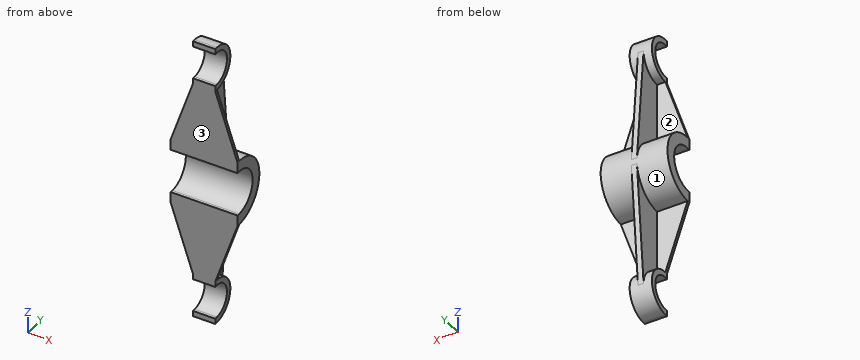
Autodesk Inventor part; units mm, degrees
ref_plane "YZ Plane" through (0, 0, 0) normal (1, 0, 0) x (0, 1, 0)
ref_plane "XZ Plane" through (0, 0, 0) normal (0, 1, 0) x (-1, 0, 0)
ref_plane "XY Plane" through (0, 0, 0) normal (0, 0, 1) x (1, 0, 0)
sketch "Boceto1" plane through (0, 0, 0) normal (1, 0, 0) x (0, 1, 0)
  arc A0 (0, -20) -> (0, 20) centre (0, 0) ccw
  arc A1 (0, -30) -> (0, 30) centre (0, 0) ccw
  line L0 (0, 0) -> (-5, 0) construction
  arc A2 (0, -125) -> (0, -95) centre (0, -110) ccw
  arc A3 (0, -130) -> (0, -90) centre (0, -110) ccw
  arc A4 (0, 95) -> (0, 125) centre (0, 110) ccw
  arc A5 (0, 90) -> (0, 130) centre (0, 110) ccw
  line L1 (0, 95) -> (-2.5, 95)
  line L2 (-2.5, 95) -> (-2.5, 90)
  line L3 (-2.5, 90) -> (0, 90)
  line L4 (0, 125) -> (-2.5, 125)
  line L5 (-2.5, 125) -> (-2.5, 130)
  line L6 (-2.5, 130) -> (0, 130)
  line L7 (0, -95) -> (-2.5, -95)
  line L8 (-2.5, -95) -> (-2.5, -90)
  line L9 (-2.5, -90) -> (0, -90)
  line L10 (0, -125) -> (-2.5, -125)
  line L11 (-2.5, -125) -> (-2.5, -130)
  line L12 (-2.5, -130) -> (0, -130)
  line L13 (0, 20) -> (-2.5, 20)
  line L14 (-2.5, 20) -> (-2.5, 30)
  line L15 (-2.5, 30) -> (0, 30)
  line L16 (0, -20) -> (-2.5, -20)
  line L17 (-2.5, -20) -> (-2.5, -30)
  line L18 (-2.5, -30) -> (0, -30)
  point P0 (0, 130)
  dimension "d0" = 20
  dimension "d1" = 30
  dimension "d2" = 5
  dimension "d3" = 15
  dimension "d5" = 20
  dimension "d6" = 110
  dimension "d7" = 2.5
  dimension "d8" = 5
  dimension "d9" = 5
  dimension "d10" = 10
  dimension "d11" = 10
  dimension "d16" = 2.5
extrude "Extrusión1" add sketch "Boceto1" along normal mid plane 60 contours A0 L13 L14 L15 A1 L18 L17 L16
extrude "Extrusión2" add sketch "Boceto1" along normal mid plane 20 contours A2 L7 L8 L9 A3 L12 L11 L10 | A4 L4 L5 L6 A5 L3 L2 L1
sketch "Boceto2" plane through (-30, -2.5, 20) normal (0, -1, 0) x (1, 0, 0)
  line L0 (40, 70) -> (20, 70)
  line L1 (40, 75) -> (40, 70)
  line L2 (60, 10) -> (40, 70)
  line L3 (0, 10) -> (60, 10)
  line L4 (20, 70) -> (0, 10)
  line L5 (60, -40) -> (60, -50)
  line L6 (60, -50) -> (40, -110)
  line L7 (20, -110) -> (0, -50)
  line L8 (0, -50) -> (60, -50)
  line L9 (60, -50) -> (0, -50)
  line L10 (60, 10) -> (60, 0)
  line L11 (60, 10) -> (0, 10)
  line L12 (20, -110) -> (40, -110)
  line L13 (40, -110) -> (20, -110)
  point P0 (30, -20)
extrude "Extrusión3" add sketch "Boceto2" against normal blind 2.5
sketch "Boceto3" plane through (0, 0, 0) normal (1, 0, 0) x (0, 1, 0)
  arc A0 (0, -130) -> (0, -90) centre (0, -110) ccw
  line L0 (20, -110) -> (29.8737, -2.7502)
  arc A1 (0, -30) -> (0, 30) centre (0, 0) ccw
  arc A2 (0, 90) -> (0, 130) centre (0, 110) ccw
  line L1 (20, 110) -> (29.9301, 2.1377)
  line L2 (0, -30) -> (0, -90)
  line L3 (0, 90) -> (0, 30)
  point P0 (29.8737, 2.7502)
extrude "Extrusión4" add sketch "Boceto3" along normal mid plane 5
properties part number "Pieza de practica 10"
Verification items for the finished model (mm, model axes). Face numbers are marked on the shaded views. A direction names the side the tool comes from. Coordinates: 2 decimals unless noted, no trailing zeros. Loops run counter-clockwise (first coordinate to the right, second up) from the corner with the lowest first, then second, coordinate; pieces in that order, holes last. Notation, with made-up numbers: (7, -39.75) -> (12, -39.75) arc R12 cw to (12, -21.75) -> close; hole circle Ø5 at (20.25, -31). An arc over 180 degrees is marked (long way). Answer in a Markdown table with one row per item.
1) Section check D-D (x = 6.5). Record the cut outline in (y, z), and give its area (3 significant figures).
The answers:
| item | result |
|---|---|
| outline | (-2.5, -130) -> (0, -130) arc R20 ccw to (0, -90) -> (0, -30) arc R30 ccw to (0, 30) -> (0, 90) arc R20 ccw to (0, 130) -> (-2.5, 130) -> (-2.5, 125) -> (0, 125) arc R15 cw to (0, 95) -> (-2.5, 95) -> (-2.5, 20) -> (0, 20) arc R20 cw to (0, -20) -> (-2.5, -20) -> (-2.5, -95) -> (0, -95) arc R15 cw to (0, -125) -> (-2.5, -125) -> close |
| area | 1,740 mm2 |
2) Scan lines: line 1 along Z through (x, y) = (-7, 0.5); line 2 along X through (y, z) = (11.5, -49); line 3 along Z through (x, y) = (12, 8). Record each from-to range of solid material in increasing order. Write a range as from..to.
The answers:
| item | result |
|---|---|
| line 1 | z = -129.99..-124.99, -95.01..-90.01, -30..-19.99, 19.99..30, 90.01..95.01, 124.99..129.99 |
| line 2 | x = -2.5..2.5 |
| line 3 | z = -28.91..-18.33, 18.33..28.91 |
3) Section check C-C (z = 62). Record the cut outline in (x, y).
The answers:
| item | result |
|---|---|
| outline | (-19.33, -2.5) -> (19.33, -2.5) -> (19.33, 0) -> (2.5, 0) -> (2.5, 24.42) -> (-2.5, 24.42) -> (-2.5, 0) -> (-19.33, 0) -> close |
4) Section check A-A (x = -22.5). Record the cut outline in (y, z), and give its area (3 significant figures).
The answers:
| item | result |
|---|---|
| outline | (-2.5, -52.5) -> (0, -52.5) -> (0, -30) arc R30 ccw to (0, 30) -> (0, 52.5) -> (-2.5, 52.5) -> (-2.5, 20) -> (0, 20) arc R20 cw to (0, -20) -> (-2.5, -20) -> close |
| area | 948 mm2 |
5) Access from +Z, -Z, +X, -X, +Y, -Y to the whole of each face (thin tool, end or side, straight path). Record for the marked faces 1, 2 and 3.
The answers:
| item | result |
|---|---|
| face 1 | +Y |
| face 2 | -X, +Y |
| face 3 | +Z, -Z, +X, -X, -Y |
6) Depth check by flat-ended pin: P1, Ø4, axis at x = 10.5, y = 20, coming from the -Z side; P2, Ø8, axis at x = 3.5, y = 7.5, coming from the +Z side; P3, Ø4, axis at x = 5, y = 26, coming from the -Z side. Enter the tip coordinate at first touch or a pass-through.
The answers:
| item | result |
|---|---|
| P1 | stops at z = -118.59 |
| P2 | stops at z = 129.69 |
| P3 | stops at z = -18 |
7) Section check B-B (y = 11). Give the number of separate pieces and of enclosed holes in the cut face, and give its area (3 significant figures).
The answers:
| item | result |
|---|---|
| separate pieces | 4 |
| enclosed holes | 0 |
| area | 2,520 mm2 |
